Geometry: final body of the model. Coordinates: model frame, mm. Face numbers are marked on the shaded views. A direction names the side the tool comes from. Coordinates: 2 decimals unless noted, no trailing zeros. Loops run counter-clockwise (first coordinate to the right, second up) from the corner with the lowest first, then second, coordinate; pieces in that order, holes last. Notation, with made-up numbers: (1.25, 18) - (53.25, 18) arc R21 ccw to (53.25, 57) - close; hole circle Ø4 at (-28, 28.25). An arc over 180 degrees is marked (long way). Put each result on its own line as item: value. Start each with the question number.
1) Section C-C on x = 5. Output: boundary loops of the cut face in (y, z).
2) Reachability of the marked faces 4 and 5 from +Z, -Z, +X, -X, +Y, -Y: full face, straight path, thin tool, end or side. Return the list, or none.
3) Section A-A on z = 9. Output: boundary loops of the cut face in (x, y) (3 decimals).
4) Contact query for flat-ended pins moving along their axis: pin 1 Ø4 at (x, y) = (-47.685, -38.5) entering from -Z; pin 2 Ø1.6 at (y, z) = (17.5, 2) entering from -X (3 decimals); pin 3 Ø1.5 at (x, y) = (-14.5, -17.5) entering from +Z; pin 4 Ø1.4 at (x, y) = (-24.5, -35) entering from +Z. Output: stop coordinate, or through.
5) Section D-D on y = 37. Output: boundary loops of the cut face in (x, z) (1 decimal).
6) Draft query along X for the marked faces 1, 2 and 3. Return one class per face: +X half, -X half, draft (parallel to the pull), parting line (faces both ways), or undercut.
7) Material intervals for line 1 along Y through (x, z) = (-24.5, 0.5) (3 decimals); line 2 along Y through (x, z) = (62.29, -0.75); line 3 along X through (y, z) = (23, 9) (3 decimals), sorted ascending. Write a range as from..to.
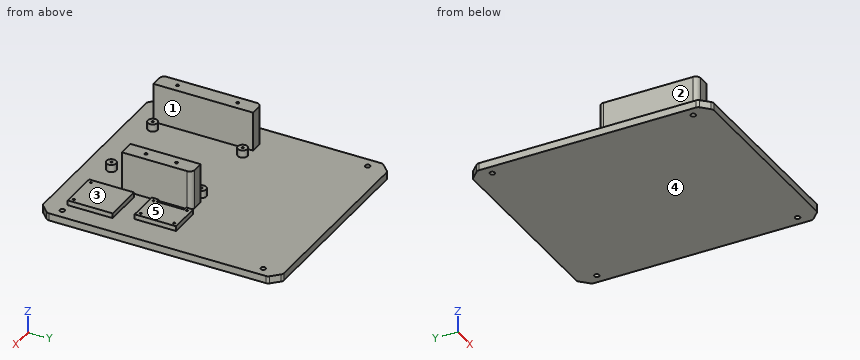
```python
from build123d import *

# Parameters (mm, degrees)
F4_W      = 136.645
F4_H      = 154.85
F5_DEPTH  = 4.7625
F0_R      = 3.1
F0_R_2    = 1.375
F6_DEPTH  = 4.7625
F7_DEPTH  = 25.4
F3_R      = 1.143
F8_DEPTH  = 3.175
F2_W      = 25.4
F2_H      = 28.956
F2_R      = 1.143
F9_DEPTH  = 3.175
F10_R     = 0.635
F11_DEPTH = 7.62
F12_R     = 0.635
F14_DEPTH = 7.62
F15_R     = 0.889
F16_DEPTH = 25.4
F17_SIZE  = 6.35
F18_R     = 2.54
F19_R     = 1.5875
F20_DEPTH = 4.7635


# Not quite as in the source:
# - a feature names something its author has since deleted; it is built from what else it names


with BuildPart() as f5:
    # F4 (on Top) → F5 (new body)
    with BuildSketch(Plane.XY):
        with Locations((14.2875, 26.225)):
            Rectangle(F4_W, F4_H)
    extrude(amount=-F5_DEPTH)

    # F0 (on Top) → F6 (join)
    with BuildSketch(Plane.XY):
        with Locations((-24.5, 23)):
            Circle(F0_R)
        with Locations((-24.5, 23)):
            Circle(F0_R_2, mode=Mode.SUBTRACT)
        with Locations((24.5, 23)):
            Circle(F0_R)
        with Locations((24.5, 23)):
            Circle(F0_R_2, mode=Mode.SUBTRACT)
        with Locations((-24.5, -35)):
            Circle(F0_R)
        with Locations((-24.5, -35)):
            Circle(F0_R_2, mode=Mode.SUBTRACT)
        with Locations((24.5, -35)):
            Circle(F0_R)
        with Locations((24.5, -35)):
            Circle(F0_R_2, mode=Mode.SUBTRACT)
        with Locations((-24.5, 23)):
            Circle(F0_R_2)
        with Locations((24.5, 23)):
            Circle(F0_R_2)
        with Locations((-24.5, -35)):
            Circle(F0_R_2)
        with Locations((24.5, -35)):
            Circle(F0_R_2)
    extrude(amount=F6_DEPTH)

    # F1 (on Top) → F7 (join)
    with BuildSketch(Plane.XY):
        with BuildLine():
            ThreePointArc((-41.335, -34.925), (-40.4050640303, -37.1700640303), (-38.16, -38.1))
            Line((-38.16, -38.1), (-34.35, -38.1))
            Line((-34.35, -38.1), (-31.175, -38.1))
            Line((-31.175, -38.1), (-31.175, -34.925))
            Line((-31.175, -34.925), (-31.175, 22.925))
            Line((-31.175, 22.925), (-31.175, 26.1))
            Line((-31.175, 26.1), (-38.16, 26.1))
            ThreePointArc((-38.16, 26.1), (-40.4050640303, 25.1700640303), (-41.335, 22.925))
            Line((-41.335, 22.925), (-41.335, -34.925))
        make_face()
        with BuildLine():
            Line((31.175, 26.1), (31.175, 22.925))
            Line((31.175, 22.925), (31.175, -19.05))
            Line((31.175, -19.05), (41.335, -19.05))
            Line((41.335, -19.05), (41.335, 22.925))
            ThreePointArc((41.335, 22.925), (40.4050640303, 25.1700640303), (38.16, 26.1))
            Line((38.16, 26.1), (31.175, 26.1))
        make_face()
    extrude(amount=F7_DEPTH)

    # F3 (on Top) → F8 (join)
    with BuildSketch(Plane.XY):
        Polygon((64.83, 28.556), (44.51, 28.556), (44.51, 24.111), (47.05, 24.111), (47.05, 6.331), (44.51, 6.331), (44.51, 1.886), (64.83, 1.886), align=None)
        with Locations((47.05, 4.426)):
            Circle(F3_R, mode=Mode.SUBTRACT)
        with Locations((62.29, 4.426)):
            Circle(F3_R, mode=Mode.SUBTRACT)
        with Locations((47.05, 26.016)):
            Circle(F3_R, mode=Mode.SUBTRACT)
        with Locations((62.29, 26.016)):
            Circle(F3_R, mode=Mode.SUBTRACT)
        with Locations((62.29, 4.426)):
            Circle(F3_R)
        with Locations((62.29, 26.016)):
            Circle(F3_R)
        with Locations((47.05, 26.016)):
            Circle(F3_R)
        with Locations((47.05, 4.426)):
            Circle(F3_R)
    extrude(amount=F8_DEPTH)

    # F2 (on Top) → F9 (join)
    with BuildSketch(Plane.XY):
        with Locations((57.21, -24.022)):
            Rectangle(F2_W, F2_H)
        with Locations((47.05, -35.96)):
            Circle(F2_R, mode=Mode.SUBTRACT)
        with Locations((67.37, -35.96)):
            Circle(F2_R, mode=Mode.SUBTRACT)
        with Locations((47.05, -35.96)):
            Circle(F2_R)
        with Locations((67.37, -35.96)):
            Circle(F2_R)
    extrude(amount=F9_DEPTH)

    # F10 (on face) → F11 (cut)
    with BuildSketch(Plane.XY.offset(3.175)):
        with Locations((47.05, 26.016)):
            Circle(F10_R)
        with Locations((62.29, 26.016)):
            Circle(F10_R)
        with Locations((62.29, 4.426)):
            Circle(F10_R)
        with Locations((47.05, 4.426)):
            Circle(F10_R)
        with Locations((47.05, -35.96)):
            Circle(F10_R)
        with Locations((67.37, -35.96)):
            Circle(F10_R)
    extrude(amount=-F11_DEPTH, mode=Mode.SUBTRACT)

    # F12 (on face) → F14 (cut)
    with BuildSketch(Plane.XY.offset(4.7625)):
        with Locations((-24.5, 23)):
            Circle(F12_R)
        with Locations((24.5, 23)):
            Circle(F12_R)
        with Locations((24.5, -35)):
            Circle(F12_R)
        with Locations((-24.5, -35)):
            Circle(F12_R)
    extrude(amount=-F14_DEPTH, mode=Mode.SUBTRACT)

    # F15 (on face) → F16 (cut)
    with BuildSketch(Plane.XY.offset(25.4)):
        with Locations((-36.255, 13.4)):
            Circle(F15_R)
        with Locations((36.255, -6.35)):
            Circle(F15_R)
        with Locations((36.255, 13.4)):
            Circle(F15_R)
        with Locations((-36.255, -25.4)):
            Circle(F15_R)
    extrude(amount=-F16_DEPTH, mode=Mode.SUBTRACT)

    # F17
    f17_edges = [f5.edges().sort_by_distance(p)[0] for p in [
        (-54.035, 103.65, -2.38125),
        (82.61, 103.65, -2.38125),
        (82.61, -51.2, -2.38125),
        (-54.035, -51.2, -2.38125),
    ]]
    chamfer(f17_edges, length=F17_SIZE)

    # F18
    f18_edges = [f5.edges().sort_by_distance(p)[0] for p in [
        (82.61, 97.3, -2.38125),
        (76.26, 103.65, -2.38125),
        (-47.685, 103.65, -2.38125),
        (-54.035, 97.3, -2.38125),
        (-54.035, -44.85, -2.38125),
        (-47.685, -51.2, -2.38125),
        (76.26, -51.2, -2.38125),
        (82.61, -44.85, -2.38125),
    ]]
    fillet(f18_edges, radius=F18_R)

    # F19 (on face) → F20 (cut, through all)
    with BuildSketch(Plane.XY):
        with Locations((-47.685, 90.95)):
            Circle(F19_R)
        with Locations((76.26, 90.95)):
            Circle(F19_R)
        with Locations((76.26, -38.5)):
            Circle(F19_R)
        with Locations((-47.685, -38.5)):
            Circle(F19_R)
    extrude(amount=-F20_DEPTH, mode=Mode.SUBTRACT)


solid = f5.part
```
Answer block:
1. outline: (-51.2, -4.76) - (103.65, -4.76) - (103.65, 0) - (-51.2, 0) - close
2. face 4: -Z, +X, -X, +Y, -Y
2. face 5: +Z, +X, +Y, -Y
3. outline: (-41.335, -34.925) arc R3.175 ccw to (-38.16, -38.1) - (-31.175, -38.1) - (-31.175, 26.1) - (-38.16, 26.1) arc R3.175 ccw to (-41.335, 22.925) - close; (31.175, -19.05) - (41.335, -19.05) - (41.335, 22.925) arc R3.175 ccw to (38.16, 26.1) - (31.175, 26.1) - close; hole circle Ø1.778 at (-36.255, -25.4); hole circle Ø1.778 at (-36.255, 13.4); hole circle Ø1.778 at (36.255, -6.35); hole circle Ø1.778 at (36.255, 13.4)
4. pin 1: stops at z = -4.76
4. pin 2: stops at x = -41.335
4. pin 3: stops at z = 0
4. pin 4: stops at z = 4.76
5. outline: (-54, -4.8) - (82.6, -4.8) - (82.6, 0) - (-54, 0) - close
6. face 1: undercut
6. face 2: -X half
6. face 3: draft
7. line 1: y = -38.1..-35.635, -34.365..-31.9, 19.9..22.365, 23.635..26.1
7. line 2: y = -51.2..3.79, 5.06..25.38, 26.65..103.65
7. line 3: x = -41.334..-31.175, 31.175..41.334
